Check sheet for the modelled part. Datum: model origin and axes. Units: mm. A direction names the side the tool comes from. Round coordinates to 2 decimals unless told otherwise and drop trailing zeros. Write each loop counter-clockwise with the first axis right and the second up, starting at its lowest first coordinate (ties: lowest second). Pieces come first, ordered by that corner, then holes. Notation, with made-up numbers: (33.25, 84.25) -> (76.25, 84.25) arc R17 cw to (76.25, 113.25) -> close; hole circle Ø5 at (-17, -1.75). An arc over 180 degrees is marked (long way). Answer as a JSON object with one key per item and string values. Group by question number.
```python
from build123d import *

# Parameters (mm, degrees)
SCHIZZO1_W                   = 16
SCHIZZO1_H                   = 61
SCHIZZO1_W_2                 = 10
SCHIZZO1_H_2                 = 55
ESTRUSIONE_ESTRUSIONE2_DEPTH = 60
RACCORDO1_R                  = 6.5
RACCORDO2_R                  = 3.25
ESTRUSIONE_ESTRUSIONE3_START = 30
ESTRUSIONE_ESTRUSIONE3_DEPTH = 30
ESTRUSIONE_ESTRUSIONE4_START = 60
ESTRUSIONE_ESTRUSIONE4_DEPTH = 60


with BuildPart() as part:
    # Schizzo1 → Estrusione-Estrusione2 (new body)
    with BuildSketch(Plane.XY):
        with Locations((-8, 30.5)):
            Rectangle(SCHIZZO1_W, SCHIZZO1_H)
        with Locations((-8, 30.5)):
            Rectangle(SCHIZZO1_W_2, SCHIZZO1_H_2, mode=Mode.SUBTRACT)
    extrude(amount=ESTRUSIONE_ESTRUSIONE2_DEPTH)

    # Raccordo1
    raccordo1_edges = [part.edges().sort_by_distance(p)[0] for p in [
        (0, 0, 30),
        (-16, 0, 30),
        (-16, 61, 30),
        (0, 61, 30),
    ]]
    fillet(raccordo1_edges, radius=RACCORDO1_R)

    # Raccordo2
    raccordo2_edges = [part.edges().sort_by_distance(p)[0] for p in [
        (-3, 3, 30),
        (-3, 58, 30),
        (-13, 58, 30),
        (-13, 3, 30),
    ]]
    fillet(raccordo2_edges, radius=RACCORDO2_R)

    # Schizzo2 → Estrusione-Estrusione3 (add)
    with BuildSketch(Plane.XY.offset(60).offset(ESTRUSIONE_ESTRUSIONE3_START)):
        with BuildLine():
            Line((-16, 14.5), (-16, 54.5))
            ThreePointArc((-16, 54.5), (-14.096194078, 59.096194078), (-9.5, 61))
            Line((-9.5, 61), (-6.5, 61))
            ThreePointArc((-6.5, 61), (-1.903805922, 59.096194078), (0, 54.5))
            Line((0, 54.5), (0, 14.5))
            Line((0, 14.5), (-3, 14.5))
            Line((-3, 14.5), (-3, 54.5))
            ThreePointArc((-3, 54.5), (-3.937792073, 56.888121647), (-6.25, 58))
            Line((-6.25, 58), (-9.75, 58))
            ThreePointArc((-9.75, 58), (-12.062207927, 56.888121647), (-13, 54.5))
            Line((-13, 54.5), (-13, 14.5))
            Line((-13, 14.5), (-16, 14.5))
        make_face()
    extrude(amount=-ESTRUSIONE_ESTRUSIONE3_DEPTH)

    # Schizzo3 → Estrusione-Estrusione4 (add)
    with BuildSketch(Plane.XY.offset(90).offset(ESTRUSIONE_ESTRUSIONE4_START)):
        with BuildLine():
            Line((-16, 6.5), (-16, 54.5))
            ThreePointArc((-16, 54.5), (-14.096194078, 59.096194078), (-9.5, 61))
            Line((-9.5, 61), (-6.5, 61))
            ThreePointArc((-6.5, 61), (-1.903805922, 59.096194078), (0, 54.5))
            Line((0, 54.5), (0, 6.5))
            ThreePointArc((0, 6.5), (-1.903805922, 1.903805922), (-6.5, 0))
            Line((-6.5, 0), (-9.5, 0))
            ThreePointArc((-9.5, 0), (-14.096194078, 1.903805922), (-16, 6.5))
        make_face()
        with BuildLine():
            Line((-13, 54.5), (-13, 6.25))
            ThreePointArc((-13, 6.25), (-12.048097039, 3.951902961), (-9.75, 3))
            Line((-9.75, 3), (-6.25, 3))
            ThreePointArc((-6.25, 3), (-3.951902961, 3.951902961), (-3, 6.25))
            Line((-3, 6.25), (-3, 54.5))
            ThreePointArc((-3, 54.5), (-3.937792073, 56.888121647), (-6.25, 58))
            Line((-6.25, 58), (-9.75, 58))
            ThreePointArc((-9.75, 58), (-12.062207927, 56.888121647), (-13, 54.5))
        make_face(mode=Mode.SUBTRACT)
    extrude(amount=-ESTRUSIONE_ESTRUSIONE4_DEPTH)


solid = part.part
```
(1) Release check for a two-part mould opening along Y. For faces 6 (the flat face through (0, 31, 76)), 7 (the flat face through (-8, 3, 120)), 8 (the cylindrical face through (-14.146, 1.955, 30.42)), 9 (the cylindrical face through (-12.023, 57.073, 30.42)) record: pulls with the +Y half, pulls with the -Y half, needs draft (parallel to the pull), parting line crosses it, or undercut.
(2) Section check B-B on y = 38.5. Record the cut outline in (x, z).
(3) Section check A-A on z = 28. Record the cut outline in (x, y), then the cut area to 3 significant figures.
(4) Section check D-D on z = 127.5. Record the cut outline in (x, y).
(5) Section check C-C on z = 76. Record the cut outline in (x, y), then the cut area to 3 significant figures.
(6) Go/stop test with flat-tipped pins: pin 1 Ø5 at (x, z) = (-2.5, 17.5) entering from -Y; pin 2 Ø1 at (x, y) = (-4.5, 56) entering from -Z; pin 3 Ø0.9 at (x, z) = (-15, 76.5) entering from -Y; pin 4 Ø1 at (x, z) = (-7.5, 69.5) entering from -Y. Record where each tip stops, or that it passes through.
(7) Access from +Z, -Z, +X, -X, +Y, -Y to the whole of each face (thin tool, end or side, straight path). Record for faces 1 (the flat face through (-1, 14.5, 75)), 2 (the flat face through (-2.8, 30.9, 0)), 3 (the cylindrical face through (-3.927, 57.023, 30.42)), 4 (the cylindrical face through (-12.023, 3.927, 30.42)), 5 (the flat face through (-8, 0, 30)).
(8) Scan lines: line 1 along X through (y, z) = (23.5, 69); line 2 along Y through (x, z) = (-7.75, 41); line 3 along Z through (x, y) = (-1.25, 4). Record each from-to range of solid material in increasing order.
Data:
{
 "1": {"face 6": "needs draft", "face 7": "undercut", "face 8": "pulls with the -Y half", "face 9": "undercut"},
 "2": {"outline": "(-16, 0) -> (-13, 0) -> (-13, 150) -> (-16, 150) -> close; (-3, 0) -> (0, 0) -> (0, 150) -> (-3, 150) -> close"},
 "3": {"outline": "(-16, 6.5) arc R6.5 ccw to (-9.5, 0) -> (-6.5, 0) arc R6.5 ccw to (0, 6.5) -> (0, 54.5) arc R6.5 ccw to (-6.5, 61) -> (-9.5, 61) arc R6.5 ccw to (-16, 54.5) -> close; hole (-13, 6.25) arc R3.25 ccw to (-9.75, 3) -> (-6.25, 3) arc R3.25 ccw to (-3, 6.25) -> (-3, 54.75) arc R3.25 ccw to (-6.25, 58) -> (-9.75, 58) arc R3.25 ccw to (-13, 54.75) -> close", "area": "399 mm²"},
 "4": {"outline": "(-16, 6.5) arc R6.5 ccw to (-9.5, 0) -> (-6.5, 0) arc R6.5 ccw to (0, 6.5) -> (0, 54.5) arc R6.5 ccw to (-6.5, 61) -> (-9.5, 61) arc R6.5 ccw to (-16, 54.5) -> close; hole (-13, 6.25) arc R3.25 ccw to (-9.75, 3) -> (-6.25, 3) arc R3.25 ccw to (-3, 6.25) -> (-3, 54.5) arc R3.51 ccw to (-6.25, 58) -> (-9.75, 58) arc R3.51 ccw to (-13, 54.5) -> close"},
 "5": {"outline": "(-16, 14.5) -> (-13, 14.5) -> (-13, 54.5) arc R3.51 cw to (-9.75, 58) -> (-6.25, 58) arc R3.51 cw to (-3, 54.5) -> (-3, 14.5) -> (0, 14.5) -> (0, 54.5) arc R6.5 ccw to (-6.5, 61) -> (-9.5, 61) arc R6.5 ccw to (-16, 54.5) -> close", "area": "296 mm²"},
 "6": {"pin 1": "stops at y = 0.18", "pin 2": "passes through", "pin 3": "stops at y = 14.5", "pin 4": "stops at y = 58"},
 "7": {"face 1": "+X, -X, -Y", "face 2": "-Z, +X, -X, +Y, -Y", "face 3": "-Z", "face 4": "+Z, -Z", "face 5": "+Z, -Z, +X, -X, -Y"},
 "8": {"line 1": "x = -16 to -13, -3 to 0", "line 2": "y = 0 to 3, 58 to 61", "line 3": "z = 0 to 60, 90 to 150"}
}
